from build123d import *

# Parameters (mm, degrees)
SKETCH2_R           = 2.413
BOSS_EXTRUDE2_DEPTH = 3.175


with BuildPart() as part:
    # Sketch2 → Boss-Extrude2 (new body)
    with BuildSketch(Plane(origin=(0, 0, 0), x_dir=(1, 0, 0), z_dir=(0, 1, 0))):
        Polygon((4.7244, 2.727633612), (0, 5.455267224), (-4.7244, 2.727633612), (-4.7244, -2.727633612), (0, -5.455267224), (4.7244, -2.727633612), align=None)
        with Locations(Location((0, 0, 0), (0, 0, 270))):
            Circle(SKETCH2_R, mode=Mode.SUBTRACT)
    extrude(amount=-BOSS_EXTRUDE2_DEPTH)

    # Sketch4 → Cut-Revolve1 (revolve, cut)
    with BuildSketch(Plane(origin=(0, 0, 0), x_dir=(0, 0, -1), z_dir=(1, 0, 0))):
        with BuildLine():
            Line((4.7244, 0), (0, 0))
            Line((0, 0), (0, 0.47939604))
            Line((0, 0.47939604), (5.455267224, 0.47939604))
            Line((5.455267224, 0.47939604), (5.455267224, -0.382883312))
            ThreePointArc((5.455267224, -0.382883312), (5.136942885, -0.101517068), (4.7244, 0))
        make_face()
        with BuildLine():
            Line((0, -3.65439604), (5.455267224, -3.65439604))
            Line((5.455267224, -3.65439604), (5.455267224, -2.792116688))
            ThreePointArc((5.455267224, -2.792116688), (5.136942885, -3.073482932), (4.7244, -3.175))
            Line((4.7244, -3.175), (0, -3.175))
            Line((0, -3.175), (0, -3.65439604))
        make_face()
    revolve(axis=Axis((0, -0.257604259, 0), (0, -1, 0)), mode=Mode.SUBTRACT)


solid = part.part
The listing builds one solid part. Answer for the finished solid, in the listing's coordinates (mm). Coordinates: 2 decimals unless noted, no trailing zeros. Write each loop counter-clockwise with the first axis right and the second up, starting at its lowest first coordinate (ties: lowest second). Pieces come first, ordered by that corner, then holes. Notation, with made-up numbers: M 39,48.25 L 45,48.25 A24 ccw 45,80.25 Z; hole C 57.25,51 d8. An arc over 180 degrees is marked long. Use one line per item in the form item = value.
Item 1: The mould has two halves that part along Z. Classify faces 1 (the face through (2, -3.175, 2)), 2 (the face through (-2.33, -1.57, -4.11)), 3 (the face through (2.33, -1.57, 4.11)), 4 (the face through (-1.468, -1.565, -1.915)): released by +Z, released by -Z, zero draft, split by the parting line, or undercut.
Model answer:
face_1 = zero draft
face_2 = released by -Z
face_3 = released by +Z
face_4 = undercut
Item 2: Find the intervals of material crossed by probe 1 along X at (y, z) = (-0.5, -0.5); probe 2 along Z at (x, y) = (1.5, -2.15); probe 3 along X at (y, z) = (-2.4, 0.75), in increasing order.
Model answer:
probe_1 = -4.72 to -2.36, 2.36 to 4.72
probe_2 = -4.59 to -1.89, 1.89 to 4.59
probe_3 = -4.72 to -2.29, 2.29 to 4.72
Item 3: Given P1, Ø1, axis at x = 2, y = -1, coming from the -Z side; P2, Ø2, axis at x = -0.5, z = 1, coming from the -Y side; P3, Ø1.5, axis at x = 2.5, y = -0.5, coming from the +Z side, each flat-ended and moving along its own axis, determine where each tip first touches the part or whether it passes through.
Model answer:
P1 = -4.59
P2 = through
P3 = 4.44
Item 4: Find section A-A, the plane y = -0.6. Give the vertices of the cut face in (x, z).
Model answer:
outline = M -4.72,-2.73 L 0,-5.46 L 4.72,-2.73 L 4.72,2.73 L 0,5.46 L -4.72,2.73 Z; hole C 0,0 d4.83
